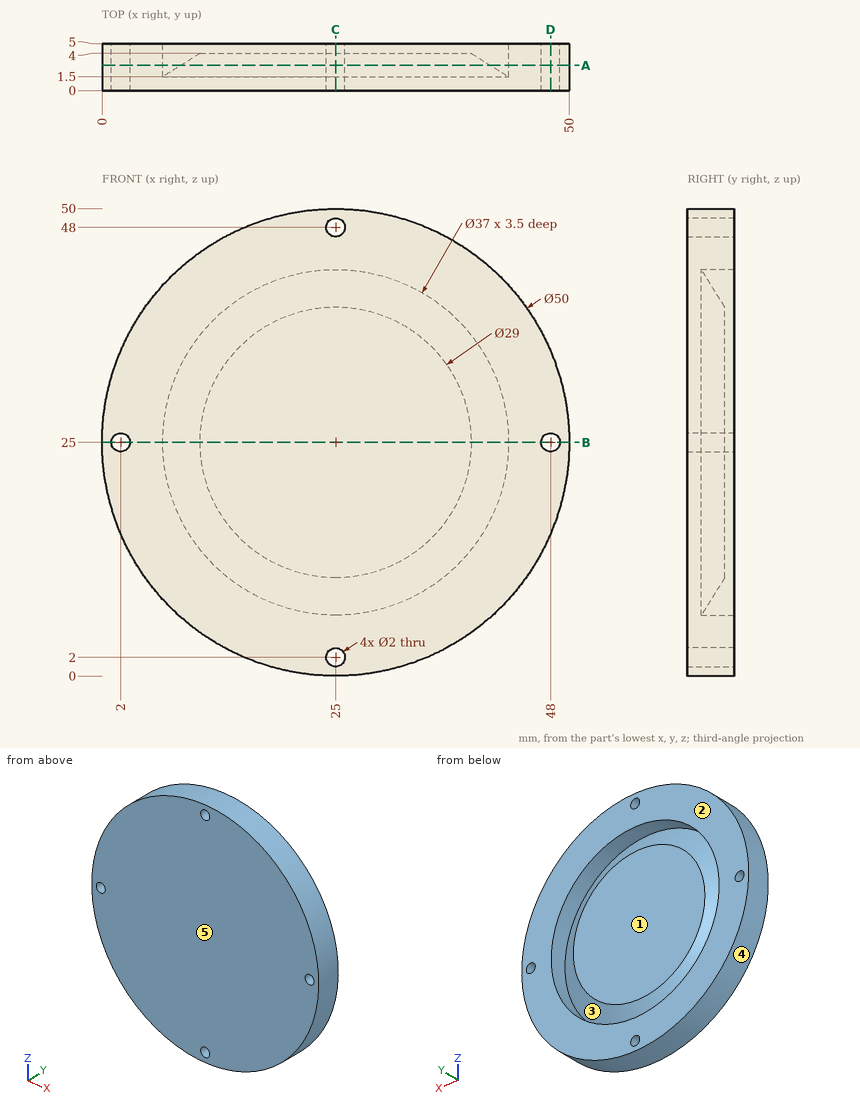
Print and shaded views of the part. All mm, measured from the part's lowest x, y and z. A direction names the side the tool comes from. Coordinates: 2 decimals unless noted, no trailing zeros. Order: outer loops, then holes, each group sorted by start corner. A loop starts at its lowest first (then second) coordinate and runs counter-clockwise, first axis right, second up. Notation, with made-up numbers: M 28.5,-31 L 46.5,-31 A24 cw 46.5,7 Z; hole C 1,30 d11. An arc over 180 degrees is marked long. Write each question's results on one line, items separated by ' | '. Start each with the question number.
Q1. Cut at B-B (z = 25). List the corners of the cut face in (x, y), then the cut area to 3 significant figures.
Q2. Drill centre lines: probe 1 along X at (y, z) = (3.7, 36); probe 2 along X at (y, z) = (1.1, 25); probe 3 along Z at (x, y) = (33.5, 2.2). Where is each one in solid material? Low to high. Write a range as from..to.
Q3. Cut at C-C (x = 25). List the corners of the cut face in (y, z).
Q4. Cut at D-D (x = 48). List the corners of the cut face in (y, z).
Q5. Flat gauge pins, fed straight in: P1, Ø14.5, axis at x = 18.5, z = 29, coming from the +Y side; P2, Ø1.2, axis at x = 48, z = 25, coming from the -Y side; P3, Ø1, axis at y = 2, z = 19.5, coming from the -X side. Where does each tip first touch, or does it go through?
Q6. Pull direction Z, two halves, no side cores. Call the marked faces 3, 4 and 5: +Z half, -Z half, draft (parallel to the pull), parting line (faces both ways), or undercut.
Q7. Cut at A-A (y = 2.7). List the corners of the cut face in (x, z).
Q8. Which spindle directions (+Z, -Z, +X, -X, +Y, -Y) get a long thin tool onto all of the face, cutting with end or side? Do the marked faces 1 and 2. Say none if no direction does.
Found:
1) outline: M 0,0 L 1,0 L 1,5 L 0,5 Z; M 3,0 L 47,0 L 47,5 L 43.5,5 L 43.5,1.5 L 39.5,4 L 10.5,4 L 6.5,1.5 L 6.5,5 L 3,5 Z; M 49,0 L 50,0 L 50,5 L 49,5 Z | area: 183 mm²
2) probe 1: 2.55..10.13, 14.83..35.17, 39.87..47.45 | probe 2: 0..1, 3..47, 49..50 | probe 3: 1.49..8.57, 9.84..40.16, 41.43..48.51
3) outline: M 0,0 L 5,0 L 5,1 L 0,1 Z; M 0,3 L 5,3 L 5,6.5 L 1.5,6.5 L 4,10.5 L 4,39.5 L 1.5,43.5 L 5,43.5 L 5,47 L 0,47 Z; M 0,49 L 5,49 L 5,50 L 0,50 Z
4) outline: M 0,15.2 L 5,15.2 L 5,24 L 0,24 Z; M 0,26 L 5,26 L 5,34.8 L 0,34.8 Z
5) P1: y = 4 | P2: through | P3: x = 0.51
6) face 3: undercut | face 4: parting line | face 5: draft
7) outline: C 25,25 d50; C 25,25 d33.16; hole C 2,25 d2; hole C 25,25 d37; hole C 25,2 d2; hole C 25,48 d2; hole C 48,25 d2
8) face 1: +Y | face 2: +Z, -Z, +X, -X, +Y
